from build123d import *

# Parameters (mm, degrees)
SKETCH1_R           = 0.77
SKETCH1_R_2         = 2
BOSS_EXTRUDE2_DEPTH = 1.25
BOSS_EXTRUDE3_START = 1.25
SKETCH1_5_R         = 0.77
SKETCH1_5_R_2       = 2
BOSS_EXTRUDE3_DEPTH = 1.25


with BuildPart() as part:
    # Sketch1 → Boss-Extrude2 (new body)
    with BuildSketch(Plane(origin=(0, 0, 0), x_dir=(1, 0, 0), z_dir=(0, 1, 0))):
        with BuildLine():
            Line((-14.242139595, -7.835793251), (-4.23908362, -7.835793251))
            ThreePointArc((-4.23908362, -7.835793251), (-0.686146993, -6.984002949), (2.094345322, -4.613819859))
            Line((2.094345322, -4.613819859), (2.026352853, 4.705737102))
            ThreePointArc((2.026352853, 4.705737102), (-0.737193213, 7.009737473), (-4.23908362, 7.835793251))
            Line((-4.23908362, 7.835793251), (-14.242139595, 7.835793251))
            ThreePointArc((-14.242139595, 7.835793251), (-22.077932846, 0), (-14.242139595, -7.835793251))
        make_face()
        with Locations(Location((-4.23908362, 0, 0), (0, 0, 270))):
            Circle(SKETCH1_R, mode=Mode.SUBTRACT)
        with Locations(Location((-14.242139595, 0, 0), (0, 0, 270))):
            Circle(SKETCH1_R_2, mode=Mode.SUBTRACT)
    extrude(amount=-BOSS_EXTRUDE2_DEPTH)

    # Sketch1_5 → Boss-Extrude3 (add)
    with BuildSketch(Plane(origin=(0, 0, 0), x_dir=(1, 0, 0), z_dir=(0, 1, 0)).offset(BOSS_EXTRUDE3_START)):
        with BuildLine():
            Line((3.27343561, 5.110155948), (3.347196034, -5))
            ThreePointArc((3.347196034, -5), (0.069203321, -7.999393891), (-4.23908362, -9.085793251))
            Line((-4.23908362, -9.085793251), (-14.242139595, -9.085793251))
            ThreePointArc((-14.242139595, -9.085793251), (-23.327932846, 0), (-14.242139595, 9.085793251))
            Line((-14.242139595, 9.085793251), (-4.23908362, 9.085793251))
            ThreePointArc((-4.23908362, 9.085793251), (0.010729233, 8.030612038), (3.27343561, 5.110155948))
        make_face()
        with Locations(Location((-4.23908362, 0, 0), (0, 0, 270))):
            Circle(SKETCH1_5_R, mode=Mode.SUBTRACT)
        with Locations(Location((-14.242139595, 0, 0), (0, 0, 270))):
            Circle(SKETCH1_5_R_2, mode=Mode.SUBTRACT)
    extrude(amount=-BOSS_EXTRUDE3_DEPTH)


solid = part.part
Verification items for the finished model (mm, model axes). A direction names the side the tool comes from. Coordinates: 2 decimals unless noted, no trailing zeros. Loops run counter-clockwise (first coordinate to the right, second up) from the corner with the lowest first, then second, coordinate; pieces in that order, holes last. Notation, with made-up numbers: (-36, -6.75) -> (8, -6.75) arc R12 ccw to (8, -1.75) -> close; hole circle Ø4 at (-40, 8). An arc over 180 degrees is marked (long way). Answer as a JSON object with one key per item and string values. Group by question number.
Item 1: Sectioned sample at D-D on y = 0.6. Record the boundary of the cut face in (x, z).
Item 2: Tool access check on faces 1 (the cylindrical face through (-0.732, -0.616, 7.007)), 2 (the flat face through (-9, -1, 7.836)), 3 (the cylindrical face through (-0.692, -0.616, -6.987)), 4 (the flat face through (-10, 0, -8)), 5 (the cylindrical face through (-22.076, -0.616, -0.172)). Record the directions out of +Z, -Z, +X, -X, +Y, -Y that give a thin tool (end or side, any length) a straight path to the whole face; none if there is none.
Item 3: Scan lines: probe 1 along X at (y, z) = (0.35, 0); probe 2 along X at (y, z) = (-0.45, 0); probe 3 along Z at (x, y) = (-12, -0.85). Record each from-to range of solid material in increasing order.
Item 4: Sectioned sample at C-C on x = -9.25. Record the boundary of the cut face in (y, z).
Item 5: Mould release check, pull along X, two halves, no side actions. Record for faces 6 (the cylindrical face through (-3.59, 0.018, 0.414)), 7 (the flat face through (-9, -1, -7.836)), 8 (the cylindrical face through (0.12, 0.63, 7.97)): +X half, -X half, draft (parallel to the pull), parting line (faces both ways), or undercut.
Item 6: Sectioned sample at B-B on z = -1.5. Record the boundary of the cut face in (x, y), plus the area to 3 significant figures.
Item 7: Depth check by flat-ended pin: pin 1 (3 mm diameter, centred on x = -14.24, z = 0, fed in from +Y); pin 2 (1.5 mm diameter, centred on y = 0, z = 3, fed in from -X). Enter the tip coordinate at first touch or a pass-through.
Item 8: Sectioned sample at A-A on y = -0.8. Record the boundary of the cut face in (x, z).
Evaluation:
{
 "1": {"outline": "(-14.24, -9.09) -> (-4.24, -9.09) arc R9.09 ccw to (3.27, -5.11) -> (3.35, 5) arc R9.09 ccw to (-4.24, 9.09) -> (-14.24, 9.09) arc R9.09 ccw to start; hole circle Ø4 at (-14.24, 0); hole circle Ø1.54 at (-4.24, 0)"},
 "2": {"face 1": "+Z, +X, -Y", "face 2": "+Z, +X, -X, -Y", "face 3": "-Z, +X, -Y", "face 4": "-Y", "face 5": "-X, -Y"},
 "3": {"probe 1": "x = -23.33 to -16.24, -12.24 to -5.01, -3.47 to 3.31", "probe 2": "x = -22.08 to -16.24, -12.24 to -5.01, -3.47 to 2.06", "probe 3": "z = -7.84 to 7.84"},
 "4": {"outline": "(-1.25, -7.84) -> (0, -7.84) -> (0, -9.09) -> (1.25, -9.09) -> (1.25, 9.09) -> (0, 9.09) -> (0, 7.84) -> (-1.25, 7.84) -> close"},
 "5": {"face 6": "undercut", "face 7": "draft", "face 8": "+X half"},
 "6": {"outline": "(-23.2, 0) -> (-21.93, 0) -> (-21.93, -1.25) -> (-15.57, -1.25) -> (-15.57, 1.25) -> (-23.2, 1.25) -> close; (-12.92, -1.25) -> (2.05, -1.25) -> (2.05, 0) -> (3.3, 0) -> (3.3, 1.25) -> (-12.92, 1.25) -> close", "area": "56.5 mm²"},
 "7": {"pin 1": "passes through", "pin 2": "stops at x = -23.04"},
 "8": {"outline": "(-14.24, -7.84) -> (-4.24, -7.84) arc R7.84 ccw to (2.03, -4.71) -> (2.09, 4.61) arc R7.84 ccw to (-4.24, 7.84) -> (-14.24, 7.84) arc R7.84 ccw to start; hole circle Ø4 at (-14.24, 0); hole circle Ø1.54 at (-4.24, 0)"}
}
